Answer from the drawing. Dimensions are ordinates in mm from the lowest x, y and z of the part. Coordinates: 2 decimals unless noted, no trailing zeros. Order: outer loops, then holes, each group sorted by start corner. A loop starts at its lowest first (then second) coordinate and runs counter-clockwise, first axis right, second up. Notation, with made-up numbers: (57, 31.25) -> (116, 31.25) arc R19 ccw to (116, 45.25) -> close; hole circle Ø1 at (71.25, 29.25). An arc over 180 degrees is marked (long way). Answer in a Markdown table with one row per item.
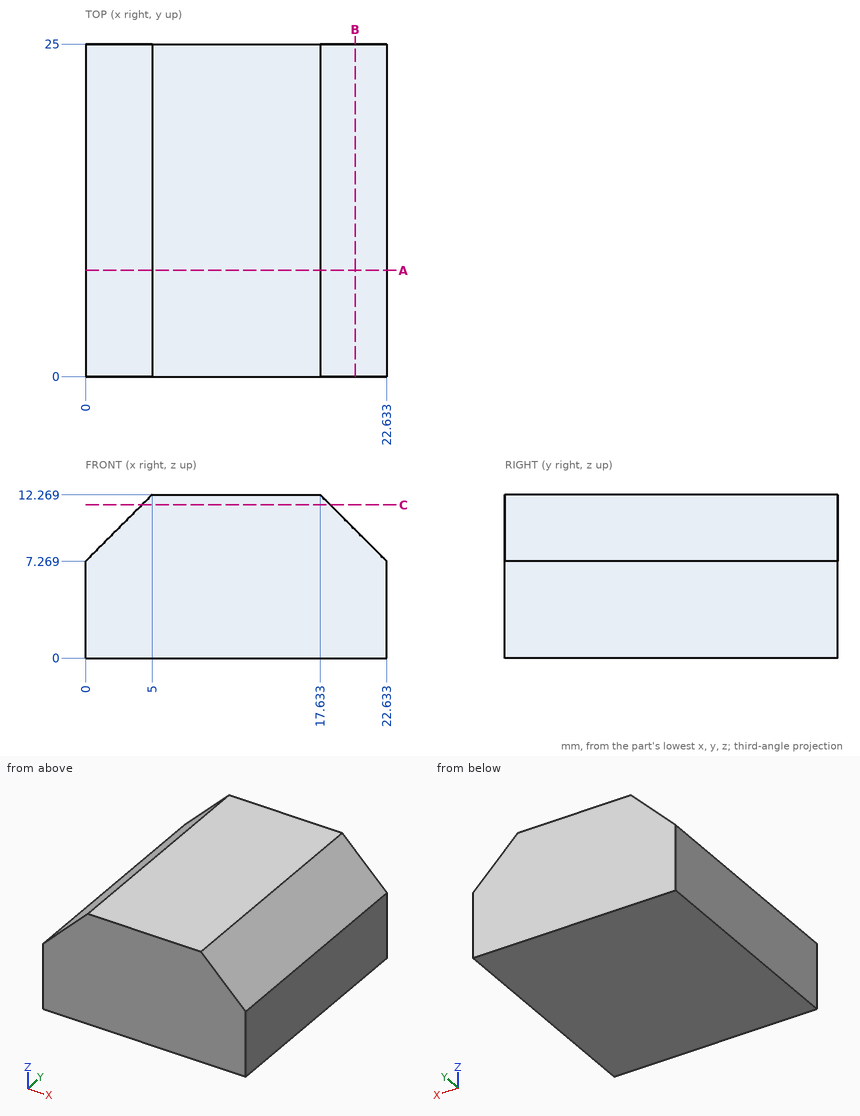
(1) A cutting plane is placed at C-C, the plane z = 11.5. Determine the outline of the cut face in (x, y).
Check values:
| item | result |
|---|---|
| outline | (4.23, 0) -> (18.4, 0) -> (18.4, 25) -> (4.23, 25) -> close |
(2) A cutting plane is placed at B-B, the plane x = 20.25. Determine the outline of the cut face in (y, z).
Check values:
| item | result |
|---|---|
| outline | (0, 0) -> (25, 0) -> (25, 9.65) -> (0, 9.65) -> close |
(3) Find the intervals of material crossed by line 1 along Z through (x, y) = (21.25, 22); line 2 along X through (y, z) = (2.5, 11); line 3 along Z through (x, y) = (2.5, 5.5), in increasing order. Write a range as from..to.
Check values:
| item | result |
|---|---|
| line 1 | 0..8.65 |
| line 2 | 3.73..18.9 |
| line 3 | 0..9.77 |
(4) A cutting plane is placed at A-A, the plane y = 8. Determine the outline of the cut face in (x, z), then the cut area to 3 significant figures.
Check values:
| item | result |
|---|---|
| outline | (0, 0) -> (22.63, 0) -> (22.63, 7.27) -> (17.63, 12.27) -> (5, 12.27) -> (0, 7.27) -> close |
| area | 253 mm² |
